Design review of the part built by this model. Coordinates are the model's own, in mm. Face numbers are marked on the shaded views. Coordinates: 2 decimals unless noted, no trailing zeros. Write each loop counter-clockwise with the first axis right and the second up, starting at its lowest first coordinate (ties: lowest second). Pieces come first, ordered by that corner, then holes. Notation, with made-up numbers: (52.5, -27.75) -> (71.5, -27.75) arc R18 ccw to (71.5, 6.25) -> close; hole circle Ø1 at (60, -10). An arc over 180 degrees is marked (long way). Answer in a Markdown table with one row per item. Add a question column.
Item 1: To check wall thickness, follow line 1 (Z direction, x = -35, y = 52); line 2 (Y direction, x = -6.5, z = 52); line 3 (X direction, y = 53.95, z = 27.5). State the ranges of each line that lie inside material, in increasing order.
Item 2: Take a section at D-D, the plane x = -35. Write out the cut boundary in (y, z), and give its area (3 significant figures).
Item 3: Clearance check with flat-ended pins moving along their axes: P1, Ø22.5, axis at y = 29.5, z = 36.5, coming from the +X side; P2, Ø5, axis at x = -40.5, y = 12.5, coming from the +Z side. State where each tip first meets the part, or that it passes through.
Item 4: Draft analysis for pull direction Y (two halves, no side actions). For the marked faces 1, 2, 3 and 4, state which applies: released by +Y, released by -Y, zero draft, split by the parting line, or undercut.
Item 5: Take a section at C-C, the plane y = 49. Write out the cut boundary in (x, z), and give its area (3 significant figures).
Item 6: Take a section at B-B, the plane z = 27.5. Write out the cut boundary in (x, y).
Item 7: Take a section at A-A, the plane y = 9.5. Write out the cut boundary in (x, z), and give its area (3 significant figures).
from build123d import *

# Parameters (mm, degrees)
SKETCH1_W           = 70
SKETCH1_H           = 55
BOSS_EXTRUDE1_DEPTH = 5
SKETCH2_W           = 5
SKETCH2_H           = 45
SKETCH2_W_2         = 5.019591865
CUT_EXTRUDE1_DEPTH  = 5
SKETCH6_W           = 60
SKETCH6_H           = 45
BOSS_EXTRUDE4_DEPTH = 50
SKETCH7_R           = 6
CUT_EXTRUDE2_DEPTH  = 70
SKETCH8_W           = 5
SKETCH8_H           = 10
BOSS_EXTRUDE5_DEPTH = 5
SKETCH9_W           = 5
SKETCH9_H           = 10
BOSS_EXTRUDE6_DEPTH = 5


with BuildPart() as part:
    # Sketch1 → Boss-Extrude1 (new body)
    with BuildSketch(Plane.XY):
        with Locations((-35, 27.5)):
            Rectangle(SKETCH1_W, SKETCH1_H)
    extrude(amount=BOSS_EXTRUDE1_DEPTH)

    # Sketch2 → Cut-Extrude1 (cut)
    with BuildSketch(Plane.XY.offset(5)):
        with Locations((-62.5, 27.5)):
            Rectangle(SKETCH2_W, SKETCH2_H)
        with Locations((-7.509795933, 27.5)):
            Rectangle(SKETCH2_W_2, SKETCH2_H)
    extrude(amount=-CUT_EXTRUDE1_DEPTH, mode=Mode.SUBTRACT)

    # Sketch6 → Boss-Extrude4 (add)
    with BuildSketch(Plane.XY.offset(5)):
        Polygon((-70, 0), (-65, 0), (-5, 0), (0, 0), (0, 55), (-5, 55), (-65, 55), (-70, 55), align=None)
        with Locations((-35, 27.5)):
            Rectangle(SKETCH6_W, SKETCH6_H, mode=Mode.SUBTRACT)
    extrude(amount=BOSS_EXTRUDE4_DEPTH)

    # Sketch7 → Cut-Extrude2 (cut)
    with BuildSketch(Plane(origin=(0, 55, 0), x_dir=(1, 0, 0), z_dir=(0, 1, 0))):
        with Locations(Location((-35, -27.5, 0), (0, 0, 90))):
            Circle(SKETCH7_R)
    extrude(amount=-CUT_EXTRUDE2_DEPTH, mode=Mode.SUBTRACT)

    # Sketch8 → Boss-Extrude5 (add)
    with BuildSketch(Plane(origin=(-10.019591865, 0, 0), x_dir=(0, 0, -1), z_dir=(1, 0, 0))):
        with Locations((-2.5, 45)):
            Rectangle(SKETCH8_W, SKETCH8_H)
    extrude(amount=BOSS_EXTRUDE5_DEPTH)

    # Sketch9 → Boss-Extrude6 (add)
    with BuildSketch(Plane.ZY.offset(60)):
        with Locations((2.5, 45)):
            Rectangle(SKETCH9_W, SKETCH9_H)
    extrude(amount=BOSS_EXTRUDE6_DEPTH)


solid = part.part
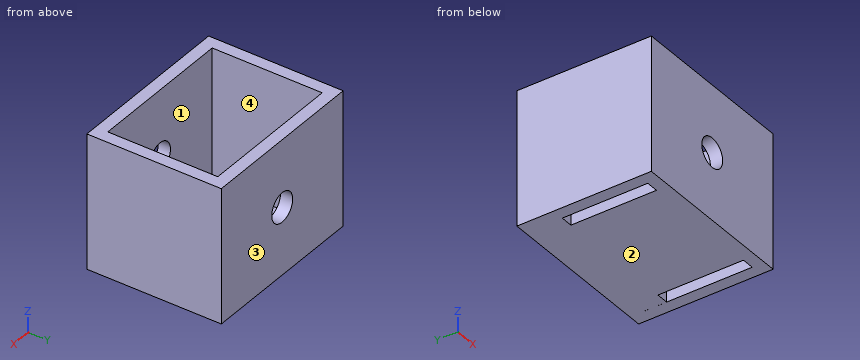
Answers:
| question | item | result |
|---|---|---|
| 1 | line 1 | z = 0 to 21.5, 33.5 to 55 |
| 1 | line 2 | y = 0 to 5, 50 to 55 |
| 1 | line 3 | x = -70 to -41, -29 to 0 |
| 2 | outline | (0, 0) -> (55, 0) -> (55, 21.5) -> (50, 21.5) -> (50, 5) -> (5, 5) -> (5, 21.5) -> (0, 21.5) -> close; (0, 33.5) -> (5, 33.5) -> (5, 55) -> (0, 55) -> close; (50, 33.5) -> (55, 33.5) -> (55, 55) -> (50, 55) -> close |
| 2 | area | 655 mm^2 |
| 3 | P1 | stops at x = 0 |
| 3 | P2 | stops at z = 5 |
| 4 | face 1 | undercut |
| 4 | face 2 | zero draft |
| 4 | face 3 | released by +Y |
| 4 | face 4 | undercut |
| 5 | outline | (-70, 0) -> (-5.02, 0) -> (-5.02, 5) -> (-65, 5) -> (-65, 55) -> (-70, 55) -> close; (-5, 0) -> (0, 0) -> (0, 55) -> (-5, 55) -> close |
| 5 | area | 850 mm^2 |
| 6 | outline | (-70, 0) -> (-41, 0) -> (-41, 5) -> (-65, 5) -> (-65, 50) -> (-41, 50) -> (-41, 55) -> (-70, 55) -> close; (-29, 0) -> (0, 0) -> (0, 55) -> (-29, 55) -> (-29, 50) -> (-5, 50) -> (-5, 5) -> (-29, 5) -> close |
| 7 | outline | (-70, 0) -> (-65, 0) -> (-65, 55) -> (-70, 55) -> close; (-60, 0) -> (-10.02, 0) -> (-10.02, 5) -> (-60, 5) -> close; (-5, 0) -> (0, 0) -> (0, 55) -> (-5, 55) -> close |
| 7 | area | 800 mm^2 |
